For this review, use the dimensioned drawing (mm, ordinates from the lowest corner) and the shaded views. Coordinates: 2 decimals unless noted, no trailing zeros. Loops run counter-clockwise (first coordinate to the right, second up) from the corner with the lowest first, then second, coordinate; pieces in that order, holes last.
1. Clearance check with a flat-ended pin moving along its axis: P1, Ø2, axis at x = 3.46, z = 3, coming from the +Y side. State where the tip first meets the part, or that it passes through.
2. To check wall thickness, follow probe 1 along X at (y, z) = (2, 3.75) (1 decimal); probe 2 along Z at (x, y) = (2.75, 8.75); probe 3 along X at (y, z) = (0.75, 4). State the ranges of each line that lie inside material, in increasing order.
3. Take a section at A-A, the plane x = 4.5. State the section outline as (y, z) points, then the cut area to 3 significant figures.
4. Take a section at C-C, the plane y = 3. State the section outline as (x, z) points, then the cut area to 3 significant figures.
5. Take a section at D-D, the plane z = 0.5. State the section outline as (x, y) points (1 decimal).
6. Mouldability with a two-part tool opening along X and no side actions: class the marked faces 1, 2 and 3 as pulls with the +X half, pulls with the -X half, needs draft (parallel to the pull), parting line crosses it, or undercut.
7. Take a section at B-B, the plane z = 2. State the section outline as (x, y) points, then the cut area to 3 significant figures.
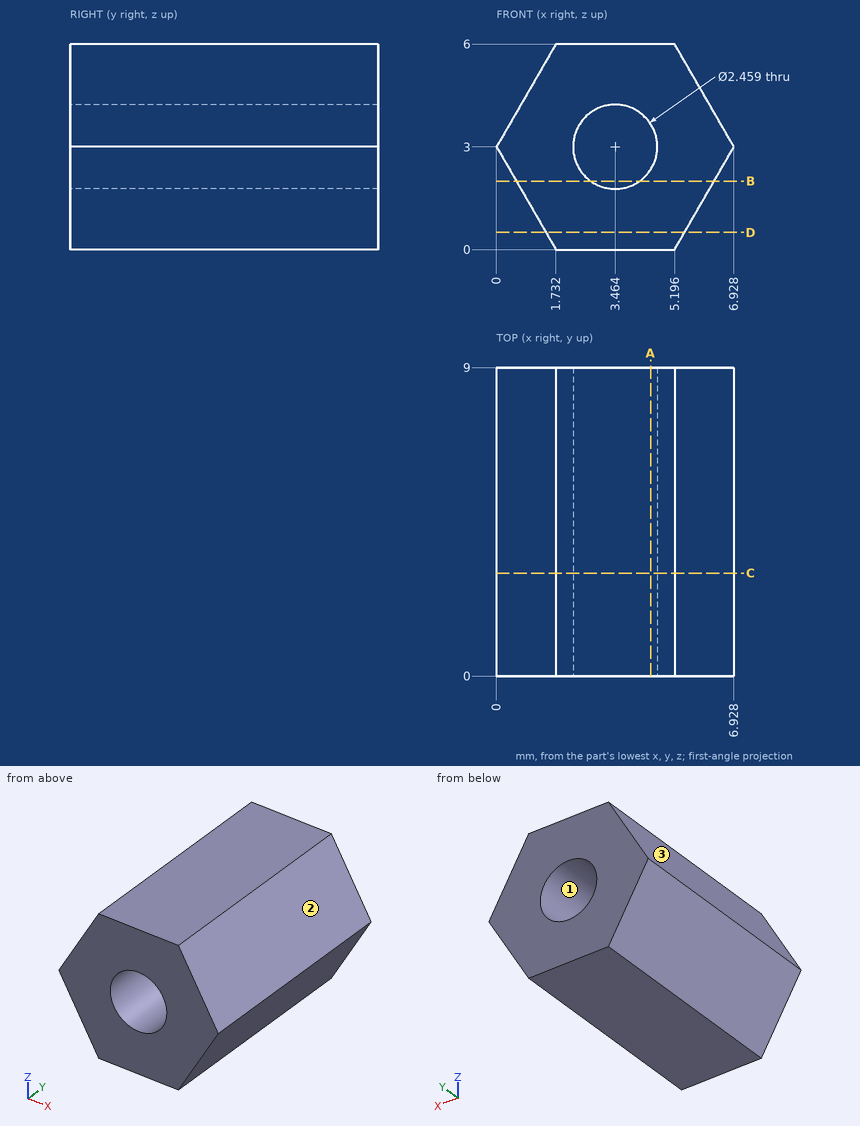
Results list:
1. P1: passes through
2. probe 1: x = 0.4 to 2.5, 4.4 to 6.5
2. probe 2: z = 0 to 2, 4 to 6
2. probe 3: x = 0.58 to 2.75, 4.18 to 6.35
3. outline: (0, 0) - (9, 0) - (9, 2.34) - (0, 2.34) - close; (0, 3.66) - (9, 3.66) - (9, 6) - (0, 6) - close
3. area: 42.1 mm2
4. outline: (0, 3) - (1.73, 0) - (5.2, 0) - (6.93, 3) - (5.2, 6) - (1.73, 6) - close; hole circle Ø2.46 at (3.46, 3)
4. area: 26.4 mm2
5. outline: (1.4, 0) - (5.5, 0) - (5.5, 9) - (1.4, 9) - close
6. face 1: undercut
6. face 2: pulls with the +X half
6. face 3: pulls with the -X half
7. outline: (0.58, 0) - (2.75, 0) - (2.75, 9) - (0.58, 9) - close; (4.18, 0) - (6.35, 0) - (6.35, 9) - (4.18, 9) - close
7. area: 39.1 mm2
